from build123d import *

# Parameters (mm, degrees)
BOSS_EXTRUDE2_DEPTH      = 9.25
M6_CLEARANCE_SLOT1_DEPTH = 25


# Read off the part's stored shape, not the designer's step: M6 Clearance Slot1
with BuildPart() as part:
    # Sketch2 → Boss-Extrude2 (new, symmetric)
    with BuildSketch(Plane.XY):
        Polygon((0, 0), (0, 8), (9, 25), (25, 25), (25, 0), align=None)
    extrude(amount=BOSS_EXTRUDE2_DEPTH, both=True)

    # M6 Clearance Slot1 outline → M6 Clearance Slot1 (cut)
    with BuildSketch(Plane.YZ):
        with BuildLine():
            Line((6.8, -3.3), (18.2, -3.3))
            ThreePointArc((18.2, -3.3), (21.5, 0), (18.2, 3.3))
            Line((18.2, 3.3), (6.8, 3.3))
            ThreePointArc((6.8, 3.3), (3.5, 0), (6.8, -3.3))
        make_face()
    extrude(amount=M6_CLEARANCE_SLOT1_DEPTH, mode=Mode.SUBTRACT)


solid = part.part
Part model, mm, in its own coordinate system. A direction names the side the tool comes from. Coordinates: 2 decimals unless noted, no trailing zeros. Loops run counter-clockwise (first coordinate to the right, second up) from the corner with the lowest first, then second, coordinate; pieces in that order, holes last. Notation, with made-up numbers: (87.5, 18.25) - (132.5, 18.25) arc R19 cw to (132.5, 23.25) - close; hole circle Ø5 at (61, 69). An arc over 180 degrees is marked (long way). Write each question's results on one line, items separated by ' | '. Start each with the question number.
Q1. Slice it at D-D on y = 13. Give the cut face in (x, z), and give its area (3 significant figures).
Q2. Which spindle directions (+Z, -Z, +X, -X, +Y, -Y) get a long thin tool onto all of the face, cutting with end or side? Do faces 4 (the flat face through (12, 12, -3.3)), 5 (the flat face through (4.437, 16.381, 4.241)). Say none if no direction does.
Q3. Drop a flat-ended pin along its axis: pin 1 Ø1.5 at (x, z) = (5.5, 5.5) entering from +Y. Give the stop position or say it passes through.
Q4. Slice it at A-A on x = 16.25. Give the cut face in (y, z), and give its area (3 significant figures).
Q5. Slice it at B-B on x = 2.25. Give the cut face in (y, z), and give its area (3 significant figures).
Q6. Slice it at C-C on z = 0. Give the cut face in (x, y).
Q7. Probe line 1 along Z through (x, y) = (14, 11.5); line 2 along Y through (x, z) = (18.25, 0.5); line 3 along Y through (x, z) = (14.75, -2.75). List the from-to ranges inside material, lowest first.
Q8. Two-plate mould, pull along Z, no slides. Class faces 1 (the flat face through (13, 13, -9.25)), 2 (the cylindrical face through (15.1, 21.5, -0.1)), 3 (the flat face through (0, 3, 0)): +Z half, -Z half, draft (parallel to the pull), parting line (faces both ways), or undercut.
Answer:
1) outline: (2.65, -9.25) - (25, -9.25) - (25, -3.3) - (2.65, -3.3) - close; (2.65, 3.3) - (25, 3.3) - (25, 9.25) - (2.65, 9.25) - close | area: 266 mm2
2) face 4: +X, -X | face 5: +Z, -Z, -X, +Y
3) pin 1: stops at y = 19.81
4) outline: (0, -9.25) - (25, -9.25) - (25, 9.25) - (0, 9.25) - close; hole (6.8, -3.3) - (18.2, -3.3) arc R3.3 ccw to (18.2, 3.3) - (6.8, 3.3) arc R3.3 ccw to start | area: 353 mm2
5) outline: (0, -9.25) - (12.25, -9.25) - (12.25, -3.3) - (6.8, -3.3) arc R3.3 cw to (6.8, 3.3) - (12.25, 3.3) - (12.25, 9.25) - (0, 9.25) - close | area: 174 mm2
6) outline: (0, 0) - (25, 0) - (25, 3.5) - (0, 3.5) - close; (7.15, 21.5) - (25, 21.5) - (25, 25) - (9, 25) - close
7) line 1: z = -9.25 to -3.3, 3.3 to 9.25 | line 2: y = 0 to 3.54, 21.46 to 25 | line 3: y = 0 to 4.98, 20.02 to 25
8) face 1: -Z half | face 2: undercut | face 3: draft
